Check sheet for the drawn part. Datum: minimum x, y, z corner. Units: mm. A direction names the side the tool comes from. Coordinates: 2 decimals unless noted, no trailing zeros. Write each loop counter-clockwise with the first axis right and the second up, starting at its lowest first coordinate (ties: lowest second). Pieces come first, ordered by that corner, then holes. Notation, with made-up numbers: (43, -1) - (90, -1) arc R13 ccw to (90, 19) - close; hole circle Ø1 at (-37.75, 50). An arc over 180 degrees is marked (long way). Use one line per item in the form item = value. Start each with the question number.
1. Cross-section at D-D on z = 76. Record the boundary of the cut face in (x, y).
2. Cross-section at A-A on y = 6.25. Record the boundary of the cut face in (x, z), then the cut area to 3 significant figures.
3. Tool access check on the marked faces 1, 2 and 3. Record the directions out of +Z, -Z, +X, -X, +Y, -Y that give a thin tool (end or side, any length) a straight path to the whole face; none if there is none.
4. Go/stop test with a flat-tipped pin: pin 1 Ø24 at (x, z) = (57, 42) entering from -Y. Record where the tip stops, or that it passes through.
5. Cross-section at C-C on x = 88.5. Record the boundary of the cut face in (y, z), then the cut area to 3 significant figures.
6. Cross-section at B-B on z = 14. Record the boundary of the cut face in (x, y), then the cut area to 3 significant figures.
7. Draft check along Y on the marked faces 4, 5 and 6. Enter one of: +Y half, -Y half, draft (parallel to the pull), parting line (faces both ways), or undercut.
8. Scan lines: line 1 along Z through (x, y) = (26.5, 3.5); line 2 along Y through (x, z) = (4, 22.5); line 3 along Y through (x, z) = (52, 72.5). Record each from-to range of solid material in increasing order.
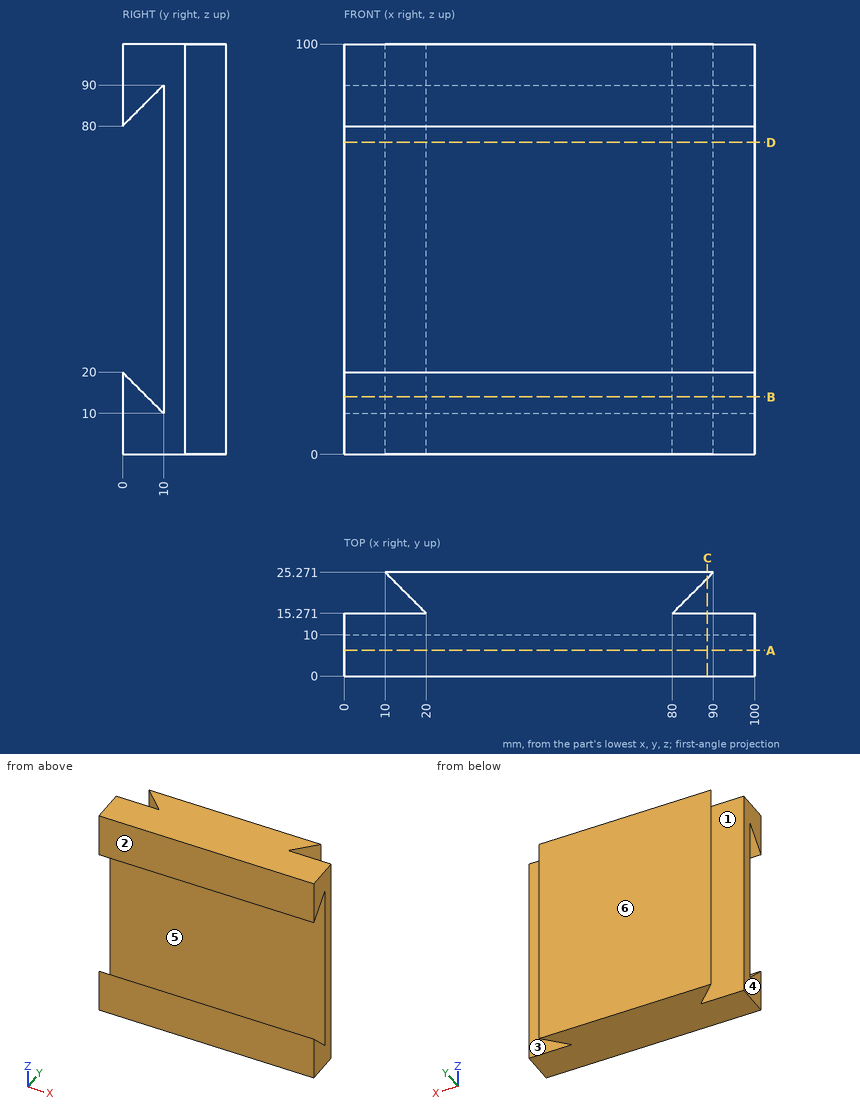
Final values:
q1.outline = (0, 10) - (100, 10) - (100, 15.27) - (80, 15.27) - (90, 25.27) - (10, 25.27) - (20, 15.27) - (0, 15.27) - close
q2.outline = (0, 0) - (100, 0) - (100, 13.75) - (0, 13.75) - close; (0, 86.25) - (100, 86.25) - (100, 100) - (0, 100) - close
q2.area = 2,750 mm²
q3.face_1 = +Z, -Z, -X
q3.face_2 = +Z, -Z, +X, -X, -Y
q3.face_3 = +Z, -Z, +X
q4.pin_1 = 10
q5.outline = (0, 0) - (15.27, 0) - (15.27, 100) - (0, 100) - (0, 80) - (10, 90) - (10, 10) - (0, 20) - close; (23.77, 0) - (25.27, 0) - (25.27, 100) - (23.77, 100) - close
q5.area = 977 mm²
q6.outline = (0, 0) - (100, 0) - (100, 6) - (0, 6) - close; (0, 10) - (100, 10) - (100, 15.27) - (80, 15.27) - (90, 25.27) - (10, 25.27) - (20, 15.27) - (0, 15.27) - close
q6.area = 1,830 mm²
q7.face_4 = draft
q7.face_5 = undercut
q7.face_6 = +Y half
q8.line_1 = 0 to 16.5, 83.5 to 100
q8.line_2 = 10 to 15.27
q8.line_3 = 10 to 25.27
